Build history of the part. All positions in model axes, mm. Face numbers are marked on the shaded views. Coordinates: 2 decimals unless noted, no trailing zeros. Order: outer loops, then holes, each group sorted by start corner. A loop starts at its lowest first (then second) coordinate and runs counter-clockwise, first axis right, second up. Notation, with made-up numbers: (30, 10.5) - (54, 10.5) arc R30 ccw to (54, 33.5) - close; hole circle Ø9 at (71.25, 2). An arc over 180 degrees is marked (long way). Return JSON: item names as keys, results as strings.
Autodesk Inventor part; units mm, degrees
ref_plane "YZ Plane" through (0, 0, 0) normal (1, 0, 0) x (0, 1, 0)
ref_plane "XZ Plane" through (0, 0, 0) normal (0, 1, 0) x (-1, 0, 0)
ref_plane "XY Plane" through (0, 0, 0) normal (0, 0, 1) x (1, 0, 0)
sketch "Sketch1" plane through (0, 0, 0) normal (0, 0, 1) x (1, 0, 0)
  line L0 (0.9375, -2.1467) -> (0.9375, -2.2475)
  arc A0 (0.9375, -2.2475) -> (4.0625, -2.2475) centre (2.5, -2.2475) ccw
  line L1 (4.0625, -2.2475) -> (4.0625, -2.1467)
  arc A1 (4.4792, -1.73) -> (4.0625, -2.1467) centre (4.4792, -2.1467) ccw
  line L2 (4.4792, -1.73) -> (5.5208, -1.73)
  arc A2 (5.9375, -2.1467) -> (5.5208, -1.73) centre (5.5208, -2.1467) ccw
  line L3 (5.9375, -2.1467) -> (5.9375, -2.2475)
  arc A3 (5.9375, -2.2475) -> (9.0625, -2.2475) centre (7.5, -2.2475) ccw
  line L4 (9.0625, -2.2475) -> (9.0625, -2.1467)
  arc A4 (9.4792, -1.73) -> (9.0625, -2.1467) centre (9.4792, -2.1467) ccw
  line L5 (9.4792, -1.73) -> (10.5208, -1.73)
  arc A5 (10.9375, -2.1467) -> (10.5208, -1.73) centre (10.5208, -2.1467) ccw
  line L6 (10.9375, -2.1467) -> (10.9375, -2.2475)
  arc A6 (10.9375, -2.2475) -> (14.0625, -2.2475) centre (12.5, -2.2475) ccw
  line L7 (14.0625, -2.2475) -> (14.0625, -2.1467)
  arc A7 (14.4792, -1.73) -> (14.0625, -2.1467) centre (14.4792, -2.1467) ccw
  line L8 (14.4792, -1.73) -> (15.5208, -1.73)
  arc A8 (15.9375, -2.1467) -> (15.5208, -1.73) centre (15.5208, -2.1467) ccw
  line L9 (15.9375, -2.1467) -> (15.9375, -2.2475)
  arc A9 (15.9375, -2.2475) -> (19.0625, -2.2475) centre (17.5, -2.2475) ccw
  line L10 (19.0625, -2.2475) -> (19.0625, -2.1467)
  arc A10 (19.4792, -1.73) -> (19.0625, -2.1467) centre (19.4792, -2.1467) ccw
  line L11 (19.4792, -1.73) -> (20.5208, -1.73)
  arc A11 (20.9375, -2.1467) -> (20.5208, -1.73) centre (20.5208, -2.1467) ccw
  line L12 (20.9375, -2.1467) -> (20.9375, -2.2475)
  arc A12 (20.9375, -2.2475) -> (24.0625, -2.2475) centre (22.5, -2.2475) ccw
  line L13 (24.0625, -2.2475) -> (24.0625, -2.1467)
  arc A13 (24.4792, -1.73) -> (24.0625, -2.1467) centre (24.4792, -2.1467) ccw
  line L14 (24.4792, -1.73) -> (25.5208, -1.73)
  arc A14 (25.9375, -2.1467) -> (25.5208, -1.73) centre (25.5208, -2.1467) ccw
  line L15 (25.9375, -2.1467) -> (25.9375, -2.2475)
  arc A15 (25.9375, -2.2475) -> (29.0625, -2.2475) centre (27.5, -2.2475) ccw
  line L16 (29.0625, -2.2475) -> (29.0625, -2.1467)
  arc A16 (29.4792, -1.73) -> (29.0625, -2.1467) centre (29.4792, -2.1467) ccw
  line L17 (29.4792, -1.73) -> (30, -1.73)
  line L18 (30, -1.73) -> (30, 0)
  line L19 (30, 0) -> (0, 0)
  line L20 (0, 0) -> (0, -1.73)
  line L21 (0, -1.73) -> (0.5208, -1.73)
  arc A17 (0.9375, -2.1467) -> (0.5208, -1.73) centre (0.5208, -2.1467) ccw
  point P0 (25, 0)
extrude "Extrusion1" add sketch "Sketch1" against normal blind 15
properties part number "520-5M-15" material "Nylon 6/6"
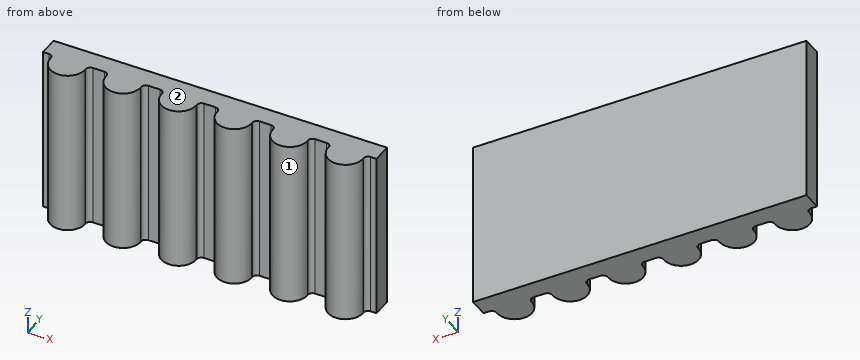
1. Cut at A-A on y = -3.1. Give the cut face in (x, z), plus the area to 3 significant figures.
Check values:
{"outline": "(1.19, -15) - (3.81, -15) - (3.81, 0) - (1.19, 0) - close; (6.19, -15) - (8.81, -15) - (8.81, 0) - (6.19, 0) - close; (11.19, -15) - (13.81, -15) - (13.81, 0) - (11.19, 0) - close; (16.19, -15) - (18.81, -15) - (18.81, 0) - (16.19, 0) - close; (21.19, -15) - (23.81, -15) - (23.81, 0) - (21.19, 0) - close; (26.19, -15) - (28.81, -15) - (28.81, 0) - (26.19, 0) - close", "area": "236 mm²"}
2. Cut at C-C on x = 21.5. Give the cut face in (y, z), plus the area to 3 significant figures.
Check values:
{"outline": "(-3.45, -15) - (0, -15) - (0, 0) - (-3.45, 0) - close", "area": "51.7 mm²"}
3. Drop a flat-ended pin along its axis: pin 1 (1.1 mm diameter, centred on x = 25, z = -8, fed in from -Y). Give the stop position or say it passes through.
Check values:
{"pin 1": "y = -1.73"}
4. Mould opens along X. For the marked faces 1 and 2 say: pulls with the +X half, pulls with the -X half, needs draft (parallel to the pull), parting line crosses it, or undercut.
Check values:
{"face 1": "undercut", "face 2": "needs draft"}
5. Probe L1, parallel to X at y = -2.25, z = -1; L2, parallel to X at y = -1.8, z = -5; L3, parallel to Y at x = 24.75, z = -12. List the from-to ranges inside material, lowest first.
Check values:
{"L1": "0.94 to 4.06, 5.94 to 9.06, 10.94 to 14.06, 15.94 to 19.06, 20.94 to 24.06, 25.94 to 29.06", "L2": "0.75 to 4.25, 5.75 to 9.25, 10.75 to 14.25, 15.75 to 19.25, 20.75 to 24.25, 25.75 to 29.25", "L3": "-1.73 to 0"}
6. Cut at B-B on x = 7. Give the cut face in (y, z).
Check values:
{"outline": "(-3.73, -15) - (0, -15) - (0, 0) - (-3.73, 0) - close"}
